CAD build for the part. Positions are in the model's coordinates, mm. Coordinates: 2 decimals unless noted, no trailing zeros. Order: outer loops, then holes, each group sorted by start corner. A loop starts at its lowest first (then second) coordinate and runs counter-clockwise, first axis right, second up. Notation, with made-up numbers: (-30.5, 51.25) - (17.5, 51.25) arc R25 ccw to (17.5, 82.25) - close; hole circle Ø6 at (28.25, 38.25). An arc over 180 degrees is marked (long way). Return JSON: item names as keys, results as strings.
from build123d import *

# Parameters (mm, degrees)
EXTRUDE_1_DEPTH           = 6
HOLE_WIZARD_16_5_16_5_1_D = 16.5
SKETCH_11_R               = 20
CUT_EXTRUDE_1_DEPTH       = 13
HOLE_WIZARD_2_D           = 9
HOLE_WIZARD_2_CBORE_D     = 14
HOLE_WIZARD_2_CBORE_DEPTH = 9
HOLE_WIZARD_M6_1_D        = 5
SKETCH_17_W               = 20
SKETCH_17_H               = 50
CUT_EXTRUDE_2_DEPTH       = 13
HOLE_WIZARD_M6_2_D        = 5
PATTERN_CIRCULAR_1_COUNT  = 4


with BuildPart() as part:
    # 草图1 → 凸台-拉伸1 (new body, symmetric)
    with BuildSketch(Plane.XY):
        with BuildLine():
            Line((-195, -160), (195, -160))
            ThreePointArc((195, -160), (209.142135624, -154.142135624), (215, -140))
            Line((215, -140), (215, 140))
            ThreePointArc((215, 140), (209.142135624, 154.142135624), (195, 160))
            Line((195, 160), (-195, 160))
            ThreePointArc((-195, 160), (-209.142135624, 154.142135624), (-215, 140))
            Line((-215, 140), (-215, -140))
            ThreePointArc((-215, -140), (-209.142135624, -154.142135624), (-195, -160))
        make_face()
    extrude(amount=EXTRUDE_1_DEPTH, both=True)

    # Ø16.5 (16.5) 直径孔1 (through all)
    with Locations(Plane.XY.offset(6)):
        with Locations((-175, 87.5), (175, 87.5), (175, -87.5), (-175, -87.5)):
            Hole(HOLE_WIZARD_16_5_16_5_1_D / 2)

    # 草图11 → 切除-拉伸1 (cut, through all)
    with BuildSketch(Plane.XY.offset(6)):
        Circle(SKETCH_11_R)
    extrude(amount=-CUT_EXTRUDE_1_DEPTH, mode=Mode.SUBTRACT)

    # 打孔尺寸(%根据)内六角圆柱头螺钉的类型2 (through all)
    with Locations(Plane.XY.offset(6)):
        with Locations((-122.5, 25), (-72.5, 25), (-72.5, -25), (-122.5, -25), (72.5, -25), (122.5, -25), (72.5, 25), (122.5, 25)):
            CounterBoreHole(HOLE_WIZARD_2_D / 2, HOLE_WIZARD_2_CBORE_D / 2, HOLE_WIZARD_2_CBORE_DEPTH)

    # M6 螺纹孔1 (through all)
    with Locations(Plane(origin=(0, 0, -6), x_dir=(-1, 0, 0), z_dir=(0, 0, -1))):
        with Locations((-97.5, 65), (-97.5, 125), (-97.5, -125), (-97.5, -65), (97.5, -65), (97.5, -125), (97.5, 125), (97.5, 65)):
            Hole(HOLE_WIZARD_M6_1_D / 2)

    # 草图17 → 切除-拉伸2 (cut, through all)
    with BuildSketch(Plane.XY.offset(6)):
        with Locations((-142.5, 135)):
            Rectangle(SKETCH_17_W, SKETCH_17_H)
        with Locations((142.5, 135)):
            Rectangle(SKETCH_17_W, SKETCH_17_H)
        with Locations((142.5, -135)):
            Rectangle(SKETCH_17_W, SKETCH_17_H)
        with Locations((-142.5, -135)):
            Rectangle(SKETCH_17_W, SKETCH_17_H)
    extrude(amount=-CUT_EXTRUDE_2_DEPTH, mode=Mode.SUBTRACT)

    # M6 螺纹孔2 (through all)
    with Locations(Plane(origin=(0, 35, 6), x_dir=(1, 0, 0), z_dir=(0, 0, 1))):
        with Locations((0, 0)):
            hole_wizard_m6_2 = Hole(HOLE_WIZARD_M6_2_D / 2)

    # 阵列(圆周)1: M6 螺纹孔2 ×4 about axis
    pattern_circular_1_axis = Axis((0, 0, 0), (0, 0, 1))
    for i in range(1, PATTERN_CIRCULAR_1_COUNT):
        add(hole_wizard_m6_2.rotate(pattern_circular_1_axis, i * 360 / PATTERN_CIRCULAR_1_COUNT), mode=Mode.SUBTRACT)


solid = part.part
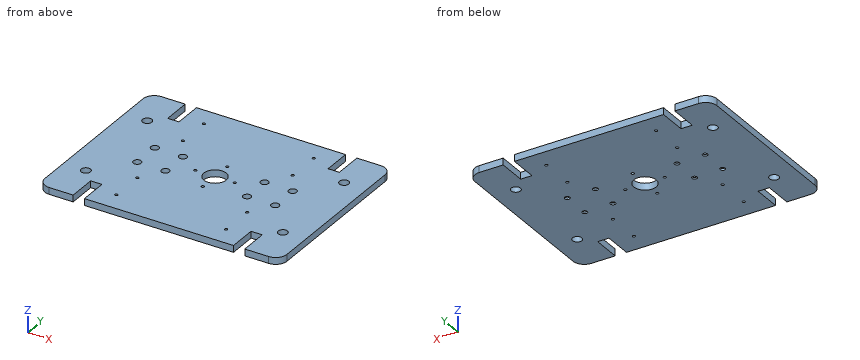
Item 1: Band-saw the part on C-C, the plane z = -0.5. Count the separate pieces of the cut face and the enclosed holes in it, then the cut area to 3 significant figures.
Findings below:
{"separate pieces": "1", "enclosed holes": "25", "area": "130,000 mm²"}
Item 2: Drop flat-ended pins along their axis: P1, Ø16, axis at x = -122.5, y = -25, coming from the +Z side; P2, Ø11.5, axis at x = 122.5, y = 25, coming from the +Z side; P3, Ø3, axis at x = -35, y = 0, coming from the -Z side. Give the stop position or say it passes through.
Findings below:
{"P1": "stops at z = 6", "P2": "stops at z = -3", "P3": "passes through"}
Item 3: Band-saw the part on A-A, the plane y = 115. List the corners of the cut face in (x, z).
Findings below:
{"outline": "(-215, -6) - (-152.5, -6) - (-152.5, 6) - (-215, 6) - close; (-132.5, -6) - (132.5, -6) - (132.5, 6) - (-132.5, 6) - close; (152.5, -6) - (215, -6) - (215, 6) - (152.5, 6) - close"}
Item 4: Band-saw the part on B-B, the plane x = -122.5. List the corners of the cut face in (y, z), then the cut area to 3 significant figures.
Findings below:
{"outline": "(-160, -6) - (-29.5, -6) - (-29.5, -3) - (-32, -3) - (-32, 6) - (-160, 6) - close; (-20.5, -6) - (20.5, -6) - (20.5, -3) - (18, -3) - (18, 6) - (-18, 6) - (-18, -3) - (-20.5, -3) - close; (29.5, -6) - (160, -6) - (160, 6) - (32, 6) - (32, -3) - (29.5, -3) - close", "area": "3,530 mm²"}
Item 5: Wall check: L1, parallel to X at y = 117, z = 0; L2, parallel to Y at x = 122.5, z = -4.4; L3, parallel to Y at x = -178, z = 2.75. Give the ranges that are in metal, low to high. Write a range as [from, to].
Findings below:
{"L1": "x = [-215, -152.5], [-132.5, 132.5], [152.5, 215]", "L2": "y = [-160, -29.5], [-20.5, 20.5], [29.5, 160]", "L3": "y = [-160, -95.19], [-79.81, 79.81], [95.19, 160]"}
